Autodesk Inventor part; units mm, degrees
ref_plane "YZ Plane" through (0, 0, 0) normal (1, 0, 0) x (0, 1, 0)
ref_plane "XZ Plane" through (0, 0, 0) normal (0, 1, 0) x (-1, 0, 0)
ref_plane "XY Plane" through (0, 0, 0) normal (0, 0, 1) x (1, 0, 0)
sketch "Sketch1" plane through (0, 0, 0) normal (0, 1, 0) x (-1, 0, 0)
  line L0 (0, 0) -> (35.56, 0)
  line L1 (35.56, 0) -> (35.56, -17.75)
  line L2 (35.56, -17.75) -> (0, -17.75)
  line L3 (0, -17.75) -> (0, 0)
  dimension "d0" = 35.56
  dimension "d1" = 17.75
extrude "Extrusion1" add sketch "Sketch1" along normal blind 1.5
sketch "Sketch2" plane through (0, 1.5, 0) normal (0, 1, 0) x (1, 0, 0)
  line L0 (0, 0) -> (0, 17.75)
  line L1 (0, 0) -> (0, 2)
  line L2 (-35.56, 17.75) -> (-35.56, 0)
  line L3 (-35.56, 0) -> (-33.56, 0)
  line L4 (-33.56, 0) -> (-33.56, 2)
  line L5 (-33.56, 2) -> (-35.56, 2)
  line L6 (-35.56, 2) -> (-35.56, 0)
  line L7 (0, 17.75) -> (-35.56, 17.75)
  line L8 (-35.56, 17.75) -> (-33.56, 17.75)
  line L9 (-33.56, 17.75) -> (-33.56, 15.75)
  line L10 (-33.56, 15.75) -> (-35.56, 15.75)
  line L11 (-35.56, 15.75) -> (-35.56, 17.75)
  line L12 (0, 17.75) -> (0, 15.75)
  line L13 (0, 15.75) -> (-33.56, 15.75)
  line L14 (-33.56, 2) -> (-33.56, 15.75)
  line L15 (-33.56, 2) -> (0, 2)
  dimension "d4" = 2
  dimension "d5" = 2
  dimension "d6" = 2
  dimension "d7" = 2
  dimension "d8" = 2
  dimension "d9" = 2
extrude "Extrusion2" add sketch "Sketch2" along normal blind 1.5 contours L15 L14 L13 L0
sketch "Sketch3" plane through (0, 0, 0) normal (1, 0, 0) x (0, 0, -1)
  line L0 (0, 0) -> (0, 1.5)
  line L1 (0, 1.5) -> (17.75, 1.5)
  line L2 (2, 1.5) -> (15.75, 1.5)
  line L3 (8.875, 1.5) -> (12.875, 1.5)
  line L4 (12.875, 1.5) -> (4.875, 1.5)
  line L5 (4.875, 1.5) -> (4.875, 4.5)
  line L6 (4.875, 4.5) -> (12.875, 4.5)
  line L7 (12.875, 4.5) -> (12.875, 1.5)
  dimension "d12" = 4
  dimension "d13" = 8
  dimension "d14" = 3
extrude "Extrusion3" add sketch "Sketch3" along normal blind 1
sketch "Sketch4" plane through (0, 0, 0) normal (-1, 0, 0) x (0, 0, 1)
  line L0 (-12.875, 3) -> (-12.875, 4.5)
  line L1 (-4.875, 4.5) -> (-4.875, 1.5)
  line L2 (-12.875, 4.5) -> (-4.875, 4.5)
  line L3 (-4.875, 4.5) -> (-4.875, 3)
  line L4 (-4.875, 3) -> (-12.875, 3)
  line L5 (-12.875, 3) -> (-12.875, 4.5)
  point P0 (0, 0)
extrude "Extrusion4" add sketch "Sketch4" along normal blind 3.4
sketch "Sketch5" plane through (1, 0, 0) normal (1, 0, 0) x (0, 0, -1)
  line L0 (4.875, 4.5) -> (4.875, 1.5)
  line L1 (4.875, 4.5) -> (5.075, 4.5)
  line L2 (5.075, 4.5) -> (5.075, 4.3)
  line L3 (5.075, 4.3) -> (4.875, 4.3)
  line L4 (4.875, 4.3) -> (4.875, 4.5)
  line L5 (12.875, 1.5) -> (12.875, 4.5)
  line L6 (12.875, 1.5) -> (12.675, 1.5)
  line L7 (12.675, 1.5) -> (12.675, 1.7)
  line L8 (12.675, 1.7) -> (12.875, 1.7)
  line L9 (12.875, 1.7) -> (12.875, 1.5)
  line L10 (12.675, 1.7) -> (5.075, 1.7)
  line L11 (5.075, 1.7) -> (5.075, 4.3)
  line L12 (5.075, 4.3) -> (12.675, 4.3)
  line L13 (12.675, 4.3) -> (12.675, 1.7)
  point P0 (0, 0)
  dimension "d19" = 0.2
  dimension "d20" = 0.2
  dimension "d21" = 0.2
  dimension "d22" = 0.2
extrude "Extrusion5" cut sketch "Sketch5" against normal blind 4 contours L12 L13 L10 L11
sketch "Sketch6" plane through (0, 1.5, 0) normal (0, 1, 0) x (1, 0, 0)
  line L0 (0, 0) -> (0, 17.75)
  line L1 (0, 0) -> (0, 1)
  line L2 (0, 1) -> (-1, 1)
  circle A0 centre (-1, 1) radius 0.5
  circle A1 centre (-3.5815, 1) radius 0.5
  circle A2 centre (-6.1631, 1) radius 0.5
  circle A3 centre (-8.7446, 1) radius 0.5
  circle A4 centre (-11.3262, 1) radius 0.5
  circle A5 centre (-13.9077, 1) radius 0.5
  circle A6 centre (-16.4892, 1) radius 0.5
  circle A7 centre (-19.0708, 1) radius 0.5
  circle A8 centre (-21.6523, 1) radius 0.5
  circle A9 centre (-24.2339, 1) radius 0.5
  circle A10 centre (-26.8154, 1) radius 0.5
  circle A11 centre (-29.3969, 1) radius 0.5
  circle A12 centre (-31.9785, 1) radius 0.5
  circle A13 centre (-34.56, 1) radius 0.5
  line L3 (-35.56, 0) -> (0, 0)
  line L4 (0, 17.75) -> (-35.56, 17.75)
  line L5 (-35.56, 0) -> (-35.56, 17.75)
  line L6 (-35.56, 17.75) -> (-35.56, 0)
  line L7 (-35.56, 8.875) -> (-37.649, 8.875)
  line L8 (0, 17.75) -> (0, 0)
  line L9 (0, 17.75) -> (0, 16.75)
  line L10 (0, 16.75) -> (-1, 16.75)
  circle A14 centre (-1, 16.75) radius 0.5
  circle A15 centre (-3.5815, 16.75) radius 0.5
  circle A16 centre (-6.1631, 16.75) radius 0.5
  circle A17 centre (-8.7446, 16.75) radius 0.5
  circle A18 centre (-11.3262, 16.75) radius 0.5
  circle A19 centre (-13.9077, 16.75) radius 0.5
  circle A20 centre (-16.4892, 16.75) radius 0.5
  circle A21 centre (-19.0708, 16.75) radius 0.5
  circle A22 centre (-21.6523, 16.75) radius 0.5
  circle A23 centre (-24.2339, 16.75) radius 0.5
  circle A24 centre (-26.8154, 16.75) radius 0.5
  circle A25 centre (-29.3969, 16.75) radius 0.5
  circle A26 centre (-31.9785, 16.75) radius 0.5
  circle A27 centre (-34.56, 16.75) radius 0.5
  line L11 (-35.56, 17.75) -> (0, 17.75)
  dimension "d25" = 1
  dimension "d26" = 1
  dimension "d27" = 1
  dimension "d30" = 2.5815
extrude "Extrusion6" cut sketch "Sketch6" against normal blind 4 contours A0 | A14 | A1 | A2 | A3 | A4 | A5 | A6 | A7 | A8 | A9 | A10 | A11 | A12 | A13 | A15 | A16 | A17 | A18 | A19 | A20 | A21 | A22 | A23 | A24 | A25 | A26 | A27
sketch "Sketch7" plane through (0, 1.5, 0) normal (0, 1, 0) x (1, 0, 0)
  line L0 (0, 2) -> (-33.56, 2)
  line L1 (-27.8322, 0.2614) -> (-18.3502, 0.2614)
  line L2 (-18.3502, 0.2614) -> (-18.3502, 2)
  line L3 (-18.3502, 2) -> (-27.8322, 2)
  line L4 (-27.8322, 2) -> (-27.8322, 0.2614)
  point P0 (0, 0)
extrude "Extrusion7" add sketch "Sketch7" against normal blind 1.5
properties part number "Teensy 3.2"
Can you work these out from the model? Positions are in its coordinate system, mm. A direction names the side the tool comes from. Round coordinates to 2 decimals unless told otherwise and drop trailing zeros. Loops run counter-clockwise (first coordinate to the right, second up) from the corner with the lowest first, then second, coordinate; pieces in that order, holes last.
Item 1: Suppose I cut it at C-C, the plane x = -34.56. Write out the boundary of the cut face in (y, z), then the cut area to 3 significant figures.
Item 2: Which directions (+Z, -Z, +X, -X, +Y, -Y) give clear straight access to the entire face, cutting with the end or side of a thin tool? Please do faces 4 (the flat face through (-33.56, 2, -9)), 5 (the flat face through (-3, 3, -9)), 6 (the cylindrical face through (-3.647, 0.76, -17.246)).
Item 3: Suppose I cut it at D-D, the plane z = -6.5. Write out the boundary of the cut face in (x, y), then the cut area to 3 significant figures.
Item 4: Suppose I cut it at B-B, the plane y = 0.7. State how many separate pieces and enclosed holes the cut face has, then the cut area to 3 significant figures.
Item 5: Suppose I cut it at A-A, the plane x = -1. Write out the boundary of the cut face in (y, z) (3 decimals).
Item 6: Will these pins go through, and if not, where does the flat tip stop? pin 1 Ø8 at (x, z) = (-18, -14) entering from +Y; pin 2 Ø0.8 at (y, z) = (3.5, -9.5) entering from +X; pin 3 Ø0.5 at (x, z) = (0.5, -8) entering from -Y.
Item 7: If we mould it in two halves opening along X, with no side actions, what happens to faces 1 (the flat face through (-1, 4.5, -9)), 2 (the flat face through (-3.4, 4, -9)), 3 (the cylindrical face through (-1.065, 0.76, -17.246))? For each: +X half, -X half, draft (parallel to the pull), parting line (faces both ways), or undercut.
Item 8: Please list where these lines run through material, in increasing order: L1, parallel to Y at x = -2, z = -10.5; L2, parallel to Y at x = -26, z = -10.25; L3, parallel to X at y = 0.3, z = -4.25.
Reported:
1. outline: (0, -17.75) - (1.5, -17.75) - (1.5, -17.25) - (0, -17.25) - close; (0, -16.25) - (1.5, -16.25) - (1.5, -1.5) - (0, -1.5) - close; (0, -0.5) - (1.5, -0.5) - (1.5, 0) - (0, 0) - close
1. area: 23.6 mm2
2. face 4: +Z, -Z, -X, +Y
2. face 5: +X
2. face 6: +Y, -Y
3. outline: (-35.56, 0) - (0, 0) - (0, 1.5) - (1, 1.5) - (1, 1.7) - (-3, 1.7) - (-3, 4.3) - (1, 4.3) - (1, 4.5) - (-3.4, 4.5) - (-3.4, 3) - (-33.56, 3) - (-33.56, 1.5) - (-35.56, 1.5) - close
3. area: 101 mm2
4. separate pieces: 1
4. enclosed holes: 24
4. area: 612 mm2
5. outline: (0, -17.75) - (1.5, -17.75) - (1.5, -17.25) - (0, -17.25) - close; (0, -16.25) - (1.5, -16.25) - (1.5, -15.75) - (3, -15.75) - (3, -12.875) - (4.5, -12.875) - (4.5, -4.875) - (3, -4.875) - (3, -2) - (1.5, -2) - (1.5, -1.5) - (0, -1.5) - close; (0, -0.5) - (1.5, -0.5) - (1.5, 0) - (0, 0) - close; hole (1.7, -12.675) - (4.3, -12.675) - (4.3, -5.075) - (1.7, -5.075) - close
6. pin 1: stops at y = 3
6. pin 2: stops at x = -3
6. pin 3: stops at y = 1.5
7. face 1: draft
7. face 2: -X half
7. face 3: undercut
8. L1: y = 0 to 1.7, 4.3 to 4.5
8. L2: y = 0 to 3
8. L3: x = -35.56 to 0
